Check sheet for the modelled part. Datum: model origin and axes. Units: mm. Face numbers are marked on the shaded views. A direction names the side the tool comes from. Round coordinates to 2 decimals unless told otherwise and drop trailing zeros. Write each loop counter-clockwise with the first axis right and the second up, starting at its lowest first coordinate (ties: lowest second). Pieces come first, ordered by that corner, then holes. Notation, with made-up numbers: M -12.75,-2.5 L 35.25,-2.5 A25 cw 35.25,31.5 Z; hole C 66,15.5 d8. An arc over 180 degrees is marked long. One line per item, written item: value.
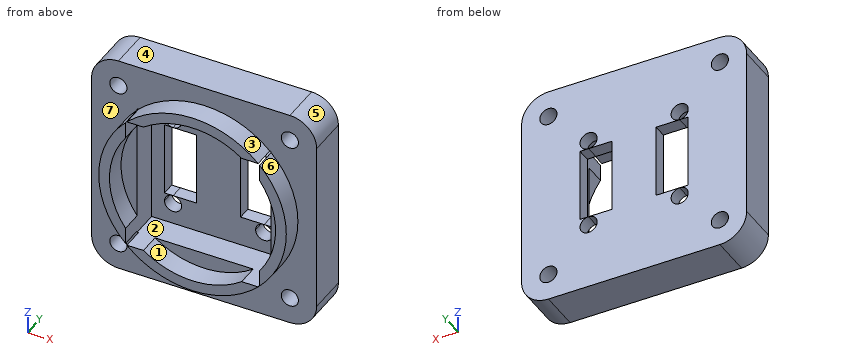
Autodesk Inventor part; units mm, degrees
ref_plane "YZ Plane" through (0, 0, 0) normal (1, 0, 0) x (0, 1, 0)
ref_plane "XZ Plane" through (0, 0, 0) normal (0, 1, 0) x (-1, 0, 0)
ref_plane "XY Plane" through (0, 0, 0) normal (0, 0, 1) x (1, 0, 0)
sketch "スケッチ1" plane through (0, 0, 0) normal (0, 1, 0) x (-1, 0, 0)
  line L0 (-5, 0) -> (-21, 0)
  line L1 (-21, -21) -> (0, -21)
  line L2 (0, -21) -> (0, -5)
  arc A0 (0, -5) -> (-5, 0) centre (-5, -5) ccw
  line L3 (0, -5) -> (0, -8)
  circle A1 centre (-5, -5) radius 1.6
  line L4 (-21, -21) -> (-8.5, -21)
  line L5 (-8.5, -21) -> (-8.5, -8.5)
  line L6 (-8.5, -8.5) -> (-21, -8.5)
  line L7 (-8.5, -8.5) -> (-8.5, -11.5)
  circle A2 centre (-12.5, -12.5) radius 1.6
  line L8 (-5, -42) -> (-21, -42)
  line L9 (0, -21) -> (0, -37)
  arc A3 (-5, -42) -> (0, -37) centre (-5, -37) ccw
  line L10 (0, -37) -> (0, -34)
  circle A4 centre (-5, -37) radius 1.6
  line L11 (-8.5, -21) -> (-8.5, -33.5)
  line L12 (-8.5, -33.5) -> (-21, -33.5)
  line L13 (-8.5, -33.5) -> (-8.5, -30.5)
  circle A5 centre (-12.5, -29.5) radius 1.6
  line L14 (-37, 0) -> (-21, 0)
  line L15 (-21, -21) -> (-42, -21)
  line L16 (-42, -21) -> (-42, -5)
  arc A6 (-37, 0) -> (-42, -5) centre (-37, -5) ccw
  line L17 (-42, -5) -> (-42, -8)
  circle A7 centre (-37, -5) radius 1.6
  line L18 (-21, -21) -> (-33.5, -21)
  line L19 (-33.5, -21) -> (-33.5, -8.5)
  line L20 (-33.5, -8.5) -> (-21, -8.5)
  line L21 (-33.5, -8.5) -> (-33.5, -11.5)
  circle A8 centre (-29.5, -12.5) radius 1.6
  circle A9 centre (-37, -37) radius 1.6
  line L22 (-42, -37) -> (-42, -34)
  line L23 (-33.5, -33.5) -> (-33.5, -30.5)
  circle A10 centre (-29.5, -29.5) radius 1.6
  line L24 (-37, -42) -> (-21, -42)
  line L25 (-42, -21) -> (-42, -37)
  line L26 (-33.5, -33.5) -> (-21, -33.5)
  line L27 (-33.5, -21) -> (-33.5, -33.5)
  arc A11 (-42, -37) -> (-37, -42) centre (-37, -37) ccw
  line L28 (-10.9, -14.1) -> (-16.9, -14.1)
  line L29 (-16.9, -14.1) -> (-16.9, -27.9)
  line L30 (-16.9, -27.9) -> (-10.9, -27.9)
  line L31 (-10.9, -27.9) -> (-10.9, -14.1)
  line L32 (-31.1, -14.1) -> (-25.1, -14.1)
  line L33 (-25.1, -14.1) -> (-25.1, -27.9)
  line L34 (-25.1, -27.9) -> (-31.1, -27.9)
  line L35 (-31.1, -27.9) -> (-31.1, -14.1)
  point P0 (0, 0)
  point P1 (0, -42)
  point P2 (-42, 0)
  point P3 (-42, -42)
  point P4 (-12.5, -14.1)
  point P5 (-12.5, -27.9)
  point P6 (-29.5, -14.1)
  point P7 (-29.5, -27.9)
  dimension "d0" = 21
  dimension "d1" = 21
  dimension "d6" = 3.2
  dimension "d7" = 12.5
  dimension "d8" = 12.5
  dimension "d9" = 3
  dimension "d11" = 3.2
  dimension "d21" = 17
  dimension "d22" = 17
  dimension "d23" = 17
  dimension "d24" = 17
  dimension "d25" = 4
  dimension "d26" = 4
  dimension "d27" = 4
  dimension "d28" = 4
  dimension "d29" = 3.2
  dimension "d30" = 3.2
  dimension "d31" = 3.2
  dimension "d32" = 2.4
  dimension "d33" = 2.4
  dimension "d34" = 6
  dimension "d35" = 6
extrude "押し出し2" add sketch "スケッチ1" against normal blind 5 contours A0 L2 L1 L5 L6 L20 L19 L15 L16 A6 L14 L0 | L9 A3 L8 L24 A11 L22 L25 L15 L27 L23 L26 L12 L11 L1
sketch "スケッチ2" plane through (0, -5, 0) normal (0, -1, 0) x (1, 0, 0)
  line L0 (33.5, -8.5) -> (8.5, -8.5)
  line L1 (8.5, -33.5) -> (33.5, -33.5)
  line L2 (33.5, -8.5) -> (8.5, -8.5)
  line L3 (8.5, -8.5) -> (8.5, -33.5)
  line L4 (8.5, -33.5) -> (33.5, -33.5)
  line L5 (33.5, -33.5) -> (33.5, -8.5)
  arc A0 (8.5, -8.7526) -> (8.5, -33.2473) centre (21.0001, -21) ccw
  arc A1 (8.5, -11.8349) -> (8.5, -30.165) centre (21.0001, -21) ccw
  arc A2 (30.1653, -8.5) -> (11.8349, -8.5) centre (21.0001, -21) ccw
  arc A3 (33.2476, -8.5) -> (8.7526, -8.5) centre (21.0001, -21) ccw
  arc A4 (11.835, -33.5) -> (30.1652, -33.5) centre (21.0001, -21) ccw
  arc A5 (33.5, -30.1652) -> (33.5, -11.8347) centre (21.0001, -21) ccw
  arc A6 (8.7527, -33.5) -> (33.2475, -33.5) centre (21.0001, -21) ccw
  arc A7 (33.5, -33.2475) -> (33.5, -8.7524) centre (21.0001, -21) ccw
  point P0 (0, 0)
  point P1 (30.1652, -33.5)
  point P2 (33.2476, -8.5)
  point P3 (8.7526, -8.5)
  point P4 (11.8349, -8.5)
extrude "押し出し4" add sketch "スケッチ1" along normal blind 2.5 contours A0 L2 L1 L5 L6 L20 L19 L15 L16 A6 L14 L0 | L9 A3 L8 L24 A11 L22 L25 L15 L27 L23 L26 L12 L11 L1 | L11 L12 L26 L23 L27 L15 L35 L34 L33 L1 L29 L30 L31 | L1 L31 L28 L29 L15 L33 L32 L35 L19 L20 L6 L5
extrude "押し出し5" add sketch "スケッチ2" along normal blind 4 contours L0 A2 A3 | A7 L5 A5 | L3 A1 A0 | A6 L1 A4
properties part number "mounter"
Q1. Sectioned sample at B-B on y = -5.75. Enter the section's corners in (x, z) (1 decimal).
Completed:
outline: M 8.5,-33.2 L 8.5,-30.2 A15.5 cw 8.5,-11.8 L 8.5,-8.8 A17.5 ccw Z; M 8.8,-33.5 A17.5 ccw 33.2,-33.5 L 30.2,-33.5 A15.5 cw 11.8,-33.5 Z; M 8.8,-8.5 L 11.8,-8.5 A15.5 cw 30.2,-8.5 L 33.2,-8.5 A17.5 ccw Z; M 33.5,-33.2 A17.5 ccw 33.5,-8.8 L 33.5,-11.8 A15.5 cw 33.5,-30.2 Z
Q2. Sectioned sample at C-C on z = -19. Enter the section's corners in (x, y), and give its area (3 significant figures).
Completed:
outline: M 0,-5 L 3.61,-5 L 3.61,-9 L 5.63,-9 L 5.63,-5 L 8.5,-5 L 8.5,0 L 10.9,0 L 10.9,2.5 L 0,2.5 Z; M 16.9,0 L 25.1,0 L 25.1,2.5 L 16.9,2.5 Z; M 31.1,0 L 33.5,0 L 33.5,-5 L 36.37,-5 L 36.37,-9 L 38.39,-9 L 38.39,-5 L 42,-5 L 42,2.5 L 31.1,2.5 Z
area: 176 mm^2
Q3. Sectioned sample at D-D on x = 21. Enter the section's corners in (y, z).
Completed:
outline: M -9,-38.5 L -5,-38.5 L -5,-42 L 2.5,-42 L 2.5,0 L -5,0 L -5,-3.5 L -9,-3.5 L -9,-5.5 L -5,-5.5 L -5,-8.5 L 0,-8.5 L 0,-33.5 L -5,-33.5 L -5,-36.5 L -9,-36.5 Z
Q4. Depth check by flat-ended pin: P1, Ø1.5, axis at y = -6, z = -33.5, coming from the -X side; P2, Ø4, axis at x = 5.5, y = -7.5, coming from the -Z side; P3, Ø3, axis at x = 37, z = -37, coming from the +Y side. Enter the tip coordinate at first touch or a pass-through.
Completed:
P1: x = 8.03
P2: z = -32.14
P3: through
Q5. Access from +Z, -Z, +X, -X, +Y, -Y to the whole of each face (thin tool, end or side, straight path). Record for the marked faces 5, 6 and 7.
Completed:
face 5: +Z, +X, +Y, -Y
face 6: +X, -Y
face 7: -Y
Q6. Draft check along X on the marked faces 1, 2, 3 and 4. Enter one of: pulls with the +X half, pulls with the -X half, needs draft (parallel to the pull), parting line crosses it, or undercut.
Completed:
face 1: undercut
face 2: undercut
face 3: parting line crosses it
face 4: needs draft
Q7. Scan lines: line 1 (X direction, y = 1.05, z = -12.5); line 2 (Z direction, x = 37, y = -2.5); line 3 (Z direction, x = 26.5, y = -1). Record each from-to range of solid material in increasing order. Write a range as [from, to].
Completed:
line 1: [0, 10.9], [14.1, 27.9], [31.1, 42]
line 2: [-42, -38.6], [-35.4, -6.6], [-3.4, 0]
line 3: [-42, -33.5], [-8.5, 0]
Q8. Sectioned sample at A-A on y = -2.75. Enter the section's corners in (x, z), and give its area (3 significant figures).
Completed:
outline: M 0,-37 A5 ccw 5,-42 L 37,-42 A5 ccw 42,-37 L 42,-5 A5 ccw 37,0 L 5,0 A5 ccw 0,-5 Z; hole C 5,-37 d3.2; hole C 5,-5 d3.2; hole M 8.5,-33.5 L 33.5,-33.5 L 33.5,-8.5 L 8.5,-8.5 Z; hole C 37,-37 d3.2; hole C 37,-5 d3.2
area: 1,090 mm^2
